```python
from build123d import *

# Parameters (mm, degrees)
CROQUIS1_W              = 18.5
CROQUIS1_H              = 5.5
SALIENTE_EXTRUIR1_DEPTH = 20
CROQUIS4_R              = 7
CORTAR_EXTRUIR1_DEPTH   = 1
CROQUIS5_W              = 30.5
CROQUIS5_H              = 8.5
SALIENTE_EXTRUIR2_DEPTH = 2
REDONDEO2_R             = 1
REDONDEO3_R             = 1
REDONDEO4_R             = 1
REDONDEO5_R             = 1
CROQUIS6_R              = 2
CORTAR_EXTRUIR2_DEPTH   = 4
REDONDEO6_R             = 1
REDONDEO7_R             = 1


with BuildPart() as part:
    # Croquis1 → Saliente-Extruir1 (new body)
    with BuildSketch(Plane.XY):
        Rectangle(CROQUIS1_W, CROQUIS1_H)
    extrude(amount=SALIENTE_EXTRUIR1_DEPTH)

    # Croquis4 → Cortar-Extruir1 (cut)
    with BuildSketch(Plane.XZ.offset(2.75)):
        with Locations((0, 11.5)):
            Circle(CROQUIS4_R)
    extrude(amount=-CORTAR_EXTRUIR1_DEPTH, mode=Mode.SUBTRACT)

    # Croquis5 → Saliente-Extruir2 (add)
    with BuildSketch(Plane.XY.offset(20)):
        Rectangle(CROQUIS5_W, CROQUIS5_H)
    extrude(amount=SALIENTE_EXTRUIR2_DEPTH)

    # Redondeo2
    redondeo2_edges = [part.edges().sort_by_distance(p)[0] for p in [
        (-15.25, 0, 22),
    ]]
    fillet(redondeo2_edges, radius=REDONDEO2_R)

    # Redondeo3
    redondeo3_edges = [part.edges().sort_by_distance(p)[0] for p in [
        (-15.25, 0, 20),
    ]]
    fillet(redondeo3_edges, radius=REDONDEO3_R - 0.0001)  # a hair under: the kernel refuses the full size

    # Redondeo4
    redondeo4_edges = [part.edges().sort_by_distance(p)[0] for p in [
        (15.25, 0, 22),
    ]]
    fillet(redondeo4_edges, radius=REDONDEO4_R)

    # Redondeo5
    redondeo5_edges = [part.edges().sort_by_distance(p)[0] for p in [
        (15.25, 0, 20),
    ]]
    fillet(redondeo5_edges, radius=REDONDEO5_R - 0.0001)  # a hair under: the kernel refuses the full size

    # Croquis6 → Cortar-Extruir2 (cut)
    with BuildSketch(Plane(origin=(0, 0, 0), x_dir=(-1, 0, 0), z_dir=(0, 0, -1))):
        Circle(CROQUIS6_R)
    extrude(amount=-CORTAR_EXTRUIR2_DEPTH, mode=Mode.SUBTRACT)

    # Redondeo6
    redondeo6_edges = [part.edges().sort_by_distance(p)[0] for p in [
        (-9.25, 0, 0),
    ]]
    fillet(redondeo6_edges, radius=REDONDEO6_R)

    # Redondeo7
    redondeo7_edges = [part.edges().sort_by_distance(p)[0] for p in [
        (9.25, 0, 0),
    ]]
    fillet(redondeo7_edges, radius=REDONDEO7_R)


solid = part.part
```
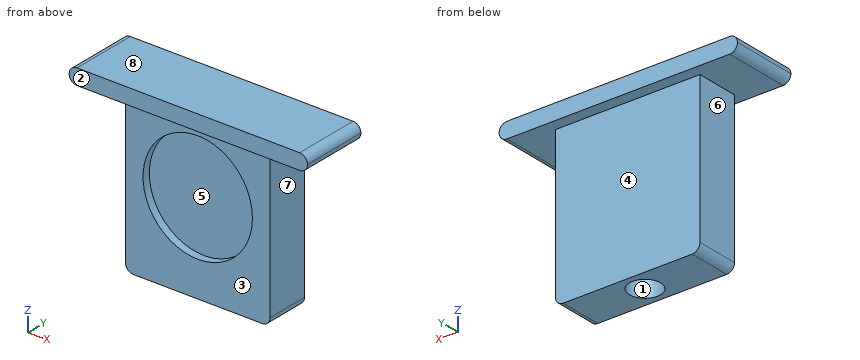
Verification items for the finished model (mm, model axes). Face numbers are marked on the shaded views. A direction names the side the tool comes from. Coordinates: 2 decimals unless noted, no trailing zeros. Loops run counter-clockwise (first coordinate to the right, second up) from the corner with the lowest first, then second, coordinate; pieces in that order, holes last. Notation, with made-up numbers: (-25, 3) -> (3, 3) arc R27 ccw to (3, 23) -> close; hole circle Ø11 at (46.5, 7). An arc over 180 degrees is marked (long way). Answer in a Markdown table with one row per item.
1) Scan lines: line 1 along Z through (x, y) = (0, -1.95); line 2 along Z through (x, y) = (5.5, 3.75); line 3 along X through (y, z) = (-1, 4.5). Record each from-to range of solid material in increasing order. Write a range as from..to.
The answers:
| item | result |
|---|---|
| line 1 | z = 4..4.5, 18.5..22 |
| line 2 | z = 20..22 |
| line 3 | x = -9.25..9.25 |
2) Section check B-B (x = 0). Record the cut outline in (y, z), and give its area (3 significant figures).
The answers:
| item | result |
|---|---|
| outline | (-4.25, 20) -> (-2.75, 20) -> (-2.75, 18.5) -> (-1.75, 18.5) -> (-1.75, 4.5) -> (-2.75, 4.5) -> (-2.75, 0) -> (-2, 0) -> (-2, 4) -> (2, 4) -> (2, 0) -> (2.75, 0) -> (2.75, 20) -> (4.25, 20) -> (4.25, 22) -> (-4.25, 22) -> close |
| area | 97.0 mm2 |
3) Section check C-C (z = 11.5). Record the cut outline in (x, y).
The answers:
| item | result |
|---|---|
| outline | (-9.25, -2.75) -> (-7, -2.75) -> (-7, -1.75) -> (7, -1.75) -> (7, -2.75) -> (9.25, -2.75) -> (9.25, 2.75) -> (-9.25, 2.75) -> close |
4) Draft check along X on the marked faces 5, 6, 7 and 8. Enter one of: released by +X, released by -X, zero draft, split by the parting line, or undercut.
The answers:
| item | result |
|---|---|
| face 5 | undercut |
| face 6 | released by -X |
| face 7 | released by +X |
| face 8 | zero draft |
5) Depth check by flat-ended pin: P1, Ø4, axis at x = -0.5, z = 12.5, coming from the -Y side; P2, Ø4, axis at y = 3, z = 17.5, coming from the -X side; P3, Ø1.5, axis at y = -0.5, z = 6.5, coming from the +X side. Enter the tip coordinate at first touch or a pass-through.
The answers:
| item | result |
|---|---|
| P1 | stops at y = -1.75 |
| P2 | stops at x = -9.25 |
| P3 | stops at x = 9.25 |
6) Access from +Z, -Z, +X, -X, +Y, -Y to the whole of each face (thin tool, end or side, straight path). Record for the marked faces 1, 2, 3 and 4.
The answers:
| item | result |
|---|---|
| face 1 | -Z |
| face 2 | +Z, -Z, +X, -X, -Y |
| face 3 | -Z, +X, -X, -Y |
| face 4 | -Z, +X, -X, +Y |
7) Section check D-D (z = 5.25). Record the cut outline in (x, y).
The answers:
| item | result |
|---|---|
| outline | (-9.25, -2.75) -> (-3.15, -2.75) -> (-3.15, -1.75) -> (3.15, -1.75) -> (3.15, -2.75) -> (9.25, -2.75) -> (9.25, 2.75) -> (-9.25, 2.75) -> close |
